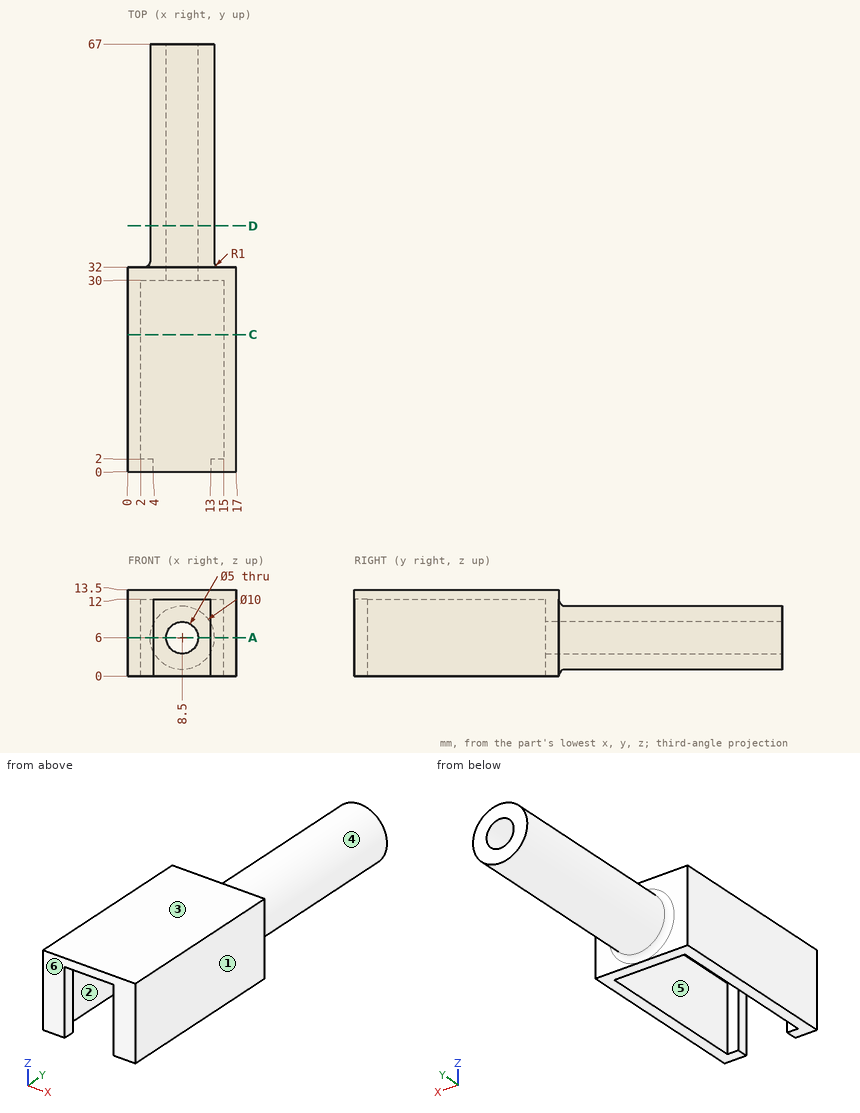
Geometry: see drawing. Coordinates: mm, zero at the bounding-box minimum. A direction names the side the tool comes from. Round coordinates to 2 decimals unless told otherwise and drop trailing zeros. Order: outer loops, then holes, each group sorted by start corner. A loop starts at its lowest first (then second) coordinate and runs counter-clockwise, first axis right, second up. Notation, with made-up numbers: (44.5, 41.25) -> (81.5, 41.25) arc R20 cw to (81.5, 79.25) -> close; hole circle Ø3 at (-15, -20.5). An arc over 180 degrees is marked (long way). Answer as CSV lines item,"result".
Item 1: Section C-C, the plane y = 21.5. Return loops of the section in (x, z), plus the area to 3 significant figures.
A:
outline,"(0, 0) -> (2, 0) -> (2, 12) -> (15, 12) -> (15, 0) -> (17, 0) -> (17, 13.5) -> (0, 13.5) -> close"
area,"73.5 mm²"
Item 2: Reachability of the marked faces 4, 5 and 6 from +Z, -Z, +X, -X, +Y, -Y: full face, straight path, thin tool, end or side. Return the list, or none.
A:
face 4,"+Y"
face 5,"-Z"
face 6,"+Z, -Z, +X, -X, -Y"
Item 3: Line query: L1, parallel to X at y = 44, z = 6; L2, parallel to Y at x = 13.5, z = 11.5; L3, parallel to X at y = 19.5, z = 11.25. Output: solid intervals per line, ascending.
A:
L1,"3.5 to 6, 11 to 13.5"
L2,"0 to 2, 30 to 32"
L3,"0 to 2, 15 to 17"
Item 4: Section D-D, the plane y = 38.5. Return loops of the section in (x, z), plus the area to 3 significant figures.
A:
outline,"circle Ø10 at (8.5, 6); hole circle Ø5 at (8.5, 6)"
area,"58.9 mm²"
Item 5: Pin query (flat end, axial travel): pin 1 Ø3 at (y, z) = (58, 4) entering from +X (3 decimals); pin 2 Ø1.5 at (y, z) = (43.5, 10.5) entering from -X; pin 3 Ø1 at (x, z) = (2.5, 6.5) entering from +Y. Return the tip coordinate at first contact, or that it passes through.
A:
pin 1,"x = 13.475"
pin 2,"x = 5.19"
pin 3,"y = 32.12"
Item 6: Section A-A, the plane z = 6. Return loops of the section in (x, y).
A:
outline,"(0, 0) -> (4, 0) -> (4, 2) -> (2, 2) -> (2, 30) -> (6, 30) -> (6, 67) -> (3.5, 67) -> (3.5, 33) arc R1 cw to (2.5, 32) -> (0, 32) -> close; (11, 30) -> (15, 30) -> (15, 2) -> (13, 2) -> (13, 0) -> (17, 0) -> (17, 32) -> (14.5, 32) arc R1 cw to (13.5, 33) -> (13.5, 67) -> (11, 67) -> close"
Item 7: Pull-direction query (X, two-part tool) for the marked faces 1, 2 and 3; classes: pulls with the +X half, pulls with the -X half, needs draft (parallel to the pull), parting line crosses it, or undercut.
A:
face 1,"pulls with the +X half"
face 2,"undercut"
face 3,"needs draft"
